Build history of the part. All positions in model axes, mm. Face numbers are marked on the shaded views. A direction names the side the tool comes from. Round coordinates to 2 decimals unless told otherwise and drop trailing zeros. Loops run counter-clockwise (first coordinate to the right, second up) from the corner with the lowest first, then second, coordinate; pieces in that order, holes last.
from build123d import *

# Parameters (mm, degrees)
F0_W     = 93.98
F0_H     = 68.58
F1_DEPTH = 45.72
F2_W     = 83.82
F2_H     = 58.42
F3_DEPTH = 41.91
F4_R     = 3.556
F4_R_2   = 1.397
F5_DEPTH = 21.59
F6_W     = 88.9
F6_H     = 63.5
F7_DEPTH = 20.32


with BuildPart() as f1:
    # F0 (on Top) → F1 (new body)
    with BuildSketch(Plane.XY):
        with Locations((-76.07475, 20.398488)):
            Rectangle(F0_W, F0_H)
    extrude(amount=F1_DEPTH)

    # F2 (on face) → F3 (cut)
    with BuildSketch(Plane.XY.offset(45.72)):
        with Locations((-76.07475, 20.398488)):
            Rectangle(F2_W, F2_H)
    extrude(amount=-F3_DEPTH, mode=Mode.SUBTRACT)

    # F4 (on face) → F5 (join)
    with BuildSketch(Plane.XY.offset(3.81)):
        with Locations((-109.09475, 43.18)):
            Circle(F4_R)
        with Locations((-109.09475, 43.18)):
            Circle(F4_R_2, mode=Mode.SUBTRACT)
        with Locations((-40.51475, 43.18)):
            Circle(F4_R)
        with Locations((-40.51475, 43.18)):
            Circle(F4_R_2, mode=Mode.SUBTRACT)
        with Locations((-109.09475, 0)):
            Circle(F4_R)
        with Locations((-109.09475, 0)):
            Circle(F4_R_2, mode=Mode.SUBTRACT)
        with Locations((-40.51475, 0)):
            Circle(F4_R)
        with Locations((-40.51475, 0)):
            Circle(F4_R_2, mode=Mode.SUBTRACT)
    extrude(amount=F5_DEPTH)

    # F6 (on face) → F7 (cut)
    with BuildSketch(Plane.XY.offset(45.72)):
        with Locations((-76.07475, 20.398488)):
            Rectangle(F6_W, F6_H)
    extrude(amount=-F7_DEPTH, mode=Mode.SUBTRACT)


solid = f1.part
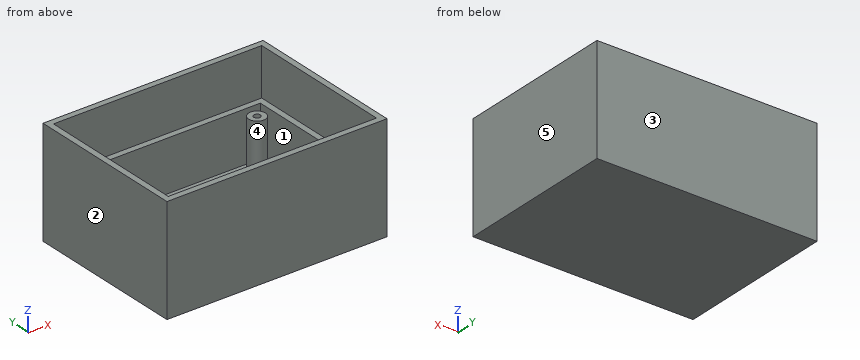
(1) Pull direction Y, two halves, no side cores. Call the marked faces 1, 2 and 3: +Y half, -Y half, draft (parallel to the pull), parting line (faces both ways), or undercut.
Responses:
face 1: undercut
face 2: draft
face 3: +Y half
(2) Slice it at C-C on y = 22. List the corners of the cut face in (x, z), plus the area to 3 significant figures.
Responses:
outline: (-123.06, 0) - (-29.08, 0) - (-29.08, 45.72) - (-31.62, 45.72) - (-31.62, 25.4) - (-34.16, 25.4) - (-34.16, 3.81) - (-117.98, 3.81) - (-117.98, 25.4) - (-120.52, 25.4) - (-120.52, 45.72) - (-123.06, 45.72) - close
area: 681 mm2
(3) Slice it at A-A on z = 12.5. Count the separate pieces of the cut face and the enclosed holes in it, plus the area to 3 significant figures.
Responses:
separate pieces: 5
enclosed holes: 5
area: 1,680 mm2
(4) Probe line 1 (X direction, y = 43, z = 16); line 2 (Y direction, x = -47, z = 21.5); line 3 (X direction, y = 47.5, z = 4). List the from-to ranges inside material, lowest first.
Responses:
line 1: x = -123.06 to -117.98, -112.65 to -110.48, -107.71 to -105.54, -44.07 to -41.9, -39.13 to -36.96, -34.16 to -29.08
line 2: y = -13.89 to -8.81, 49.61 to 54.69
line 3: x = -123.06 to -117.98, -34.16 to -29.08
(5) Which spindle directions (+Z, -Z, +X, -X, +Y, -Y) get a long thin tool onto all of the face, cutting with end or side? Do the marked faces 4 and 5. Say none if no direction does.
Responses:
face 4: +Z
face 5: +Z, -Z, +X, +Y, -Y
(6) Pin check, flat tips, straight feed: P1, Ø8, axis at x = -110.5, y = 0, coming from the +Z side; P2, Ø1.4, axis at x = -109, y = 0.5, coming from the +Z side. Stop position of each tip, or through.
Responses:
P1: stops at z = 25.4
P2: stops at z = 3.81
(7) Slice it at B-B on x = -95. List the corners of the cut face in (y, z).
Responses:
outline: (-13.89, 0) - (54.69, 0) - (54.69, 45.72) - (52.15, 45.72) - (52.15, 25.4) - (49.61, 25.4) - (49.61, 3.81) - (-8.81, 3.81) - (-8.81, 25.4) - (-11.35, 25.4) - (-11.35, 45.72) - (-13.89, 45.72) - close
(8) Slice it at D-D on y = 43.18. List the corners of the cut face in (x, z), plus the area to 3 significant figures.
Responses:
outline: (-123.06, 0) - (-29.08, 0) - (-29.08, 45.72) - (-31.62, 45.72) - (-31.62, 25.4) - (-34.16, 25.4) - (-34.16, 3.81) - (-36.96, 3.81) - (-36.96, 25.4) - (-39.12, 25.4) - (-39.12, 3.81) - (-41.91, 3.81) - (-41.91, 25.4) - (-44.07, 25.4) - (-44.07, 3.81) - (-105.54, 3.81) - (-105.54, 25.4) - (-107.7, 25.4) - (-107.7, 3.81) - (-110.49, 3.81) - (-110.49, 25.4) - (-112.65, 25.4) - (-112.65, 3.81) - (-117.98, 3.81) - (-117.98, 25.4) - (-120.52, 25.4) - (-120.52, 45.72) - (-123.06, 45.72) - close
area: 867 mm2
